Work out the finished part from the listing and answer in its coordinate system (mm). A direction names the side the tool comes from. Coordinates: 2 decimals unless noted, no trailing zeros. Write each loop counter-clockwise with the first axis right and the second up, starting at its lowest first coordinate (ties: lowest second). Pieces come first, ordered by that corner, then holes. Notation, with made-up numbers: (36, -15.5) - (75, -15.5) arc R18 cw to (75, 16.5) - close; hole circle Ø11 at (84.25, -9.5). An arc over 180 degrees is marked (long way). Use a Markdown table: item, result. Add a question column.
(1) For a pull along Y with two mould halves and no side action, classify faces 1 (the face through (2, -1.588, 2)), 2 (the face through (10.17, -2.35, 8.57)), 3 (the face through (-5.506, -2.37, -24.796)) as released by +Y, released by -Y, zero draft, split by the parting line, or undercut.
(2) Find the intervals of material crossed by line 1 (Z direction, x = 0, y = -3.4) (3 decimals); line 2 (Z direction, x = 0, y = -2) (3 decimals); line 3 (X direction, y = -0.5, z = -7), in increasing order. Write a range as from..to.
(3) Given pin 1 Ø1.6 at (x, y) = (1.5, -3) entering from +Z; pin 2 Ø2 at (y, z) = (-4, -18) entering from -X; pin 3 Ø7 at (x, z) = (-2.5, -2) entering from -Y, each flat-ended and moving along its own axis, determine where each tip first touches the part or whether it passes through.
(4) The part is cut by section D-D, the plane x = -14. Give the vertices of the cut face in (y, z) (1 decimal).
(5) The part is cut by section A-A, the plane x = 0. Give the vertices of the cut face in (y, z) (1 decimal).
(6) The part is cut by section C-C, the plane z = 15.24. Give the vertices of the cut face in (x, y) (1 decimal).
(7) The part is cut by section B-B, the plane z = 7.62. Give the vertices of the cut face in (x, y) (1 decimal).
(8) A tool of negligible diameter and unlimited length cuts with its end or side. For faces 4 (the face through (0, -3, -6.858)), 5 (the face through (24, -3.175, -10)), 6 (the face through (6, -4.762, -6)), from which of +Z, -Z, +X, -X, +Y, -Y can it reach the whole face along a straight path? Write none if from no direction.
from build123d import *

# Parameters (mm, degrees)
F0_R     = 26.67
F0_R_2   = 25.4
F1_DEPTH = 1.5875
F2_R     = 25.4
F3_DEPTH = 1.5875
F4_R     = 26.67
F4_R_2   = 25.4
F5_DEPTH = 1.5875
F6_R     = 1.905
F7_DEPTH = 25.4
F9_D     = 6.35


# Not quite as in the source:
# - a length typed as a fraction of an inch, garbled in the dataset ("3 / 203.2 mm" for 3/8 in), is restored


with BuildPart() as f1:
    # F0 (on Front) → F1 (new body)
    with BuildSketch(Plane.XZ):
        Circle(F0_R)
        Circle(F0_R_2, mode=Mode.SUBTRACT)
        Circle(F0_R_2)
        with BuildLine():
            ThreePointArc((3.9594681461, 6.858), (6.858, 3.9594681461), (7.9189362922, 0))
            ThreePointArc((7.9189362922, 0), (6.858, -3.9594681461), (3.9594681461, -6.858))
            ThreePointArc((3.9594681461, -6.858), (0, -7.9189362922), (-3.9594681461, -6.858))
            ThreePointArc((-3.9594681461, -6.858), (-6.858, -3.9594681461), (-7.9189362922, 0))
            ThreePointArc((-7.9189362922, 0), (-6.858, 3.9594681461), (-3.9594681461, 6.858))
            ThreePointArc((-3.9594681461, 6.858), (0, 7.9189362922), (3.9594681461, 6.858))
        make_face(mode=Mode.SUBTRACT)
        Polygon((3.9594681461, -6.858), (7.9189362922, 0), (3.9594681461, 6.858), (-3.9594681461, 6.858), (-7.9189362922, 0), (-3.9594681461, -6.858), align=None)
        with BuildLine():
            Line((-3.9594681461, 6.858), (3.9594681461, 6.858))
            ThreePointArc((3.9594681461, 6.858), (0, 7.9189362922), (-3.9594681461, 6.858))
        make_face()
        with BuildLine():
            Line((3.9594681461, 6.858), (7.9189362922, 0))
            ThreePointArc((7.9189362922, 0), (6.858, 3.9594681461), (3.9594681461, 6.858))
        make_face()
        with BuildLine():
            ThreePointArc((3.9594681461, -6.858), (6.858, -3.9594681461), (7.9189362922, 0))
            Line((7.9189362922, 0), (3.9594681461, -6.858))
        make_face()
        with BuildLine():
            ThreePointArc((-3.9594681461, -6.858), (0, -7.9189362922), (3.9594681461, -6.858))
            Line((3.9594681461, -6.858), (-3.9594681461, -6.858))
        make_face()
        with BuildLine():
            ThreePointArc((-7.9189362922, 0), (-6.858, -3.9594681461), (-3.9594681461, -6.858))
            Line((-3.9594681461, -6.858), (-7.9189362922, 0))
        make_face()
        with BuildLine():
            Line((-7.9189362922, 0), (-3.9594681461, 6.858))
            ThreePointArc((-3.9594681461, 6.858), (-6.858, 3.9594681461), (-7.9189362922, 0))
        make_face()
    extrude(amount=F1_DEPTH)

    # F2 (on face) → F3 (join)
    with BuildSketch(Plane.XZ.offset(1.5875)):
        Circle(F2_R)
        with BuildLine():
            ThreePointArc((3.9594681461, 6.858), (6.858, 3.9594681461), (7.9189362922, 0))
            ThreePointArc((7.9189362922, 0), (6.858, -3.9594681461), (3.9594681461, -6.858))
            ThreePointArc((3.9594681461, -6.858), (0, -7.9189362922), (-3.9594681461, -6.858))
            ThreePointArc((-3.9594681461, -6.858), (-6.858, -3.9594681461), (-7.9189362922, 0))
            ThreePointArc((-7.9189362922, 0), (-6.858, 3.9594681461), (-3.9594681461, 6.858))
            ThreePointArc((-3.9594681461, 6.858), (0, 7.9189362922), (3.9594681461, 6.858))
        make_face(mode=Mode.SUBTRACT)
        with BuildLine():
            Line((3.9594681461, 6.858), (7.9189362922, 0))
            ThreePointArc((7.9189362922, 0), (6.858, 3.9594681461), (3.9594681461, 6.858))
        make_face()
        with BuildLine():
            Line((-3.9594681461, 6.858), (3.9594681461, 6.858))
            ThreePointArc((3.9594681461, 6.858), (0, 7.9189362922), (-3.9594681461, 6.858))
        make_face()
        with BuildLine():
            Line((-7.9189362922, 0), (-3.9594681461, 6.858))
            ThreePointArc((-3.9594681461, 6.858), (-6.858, 3.9594681461), (-7.9189362922, 0))
        make_face()
        with BuildLine():
            ThreePointArc((-7.9189362922, 0), (-6.858, -3.9594681461), (-3.9594681461, -6.858))
            Line((-3.9594681461, -6.858), (-7.9189362922, 0))
        make_face()
        with BuildLine():
            ThreePointArc((-3.9594681461, -6.858), (0, -7.9189362922), (3.9594681461, -6.858))
            Line((3.9594681461, -6.858), (-3.9594681461, -6.858))
        make_face()
        with BuildLine():
            ThreePointArc((3.9594681461, -6.858), (6.858, -3.9594681461), (7.9189362922, 0))
            Line((7.9189362922, 0), (3.9594681461, -6.858))
        make_face()
    extrude(amount=F3_DEPTH)

    # F4 (on face) + F0 (on Front) → F5 (join)
    with BuildSketch(Plane.XZ.offset(3.175)):
        Circle(F4_R)
        Circle(F4_R_2, mode=Mode.SUBTRACT)
        Circle(F4_R_2)
        Polygon((7.9189362922, 0), (3.9594681461, -6.858), (-3.9594681461, -6.858), (-7.9189362922, 0), (-3.9594681461, 6.858), (3.9594681461, 6.858), align=None, mode=Mode.SUBTRACT)
    with BuildSketch(Plane.XZ):
        Circle(F0_R)
        Circle(F0_R_2, mode=Mode.SUBTRACT)
    extrude(amount=F5_DEPTH)

    # F6 (on face) → F7 (cut)
    with BuildSketch(Plane.XZ.offset(1.5875)):
        Circle(F6_R)
    extrude(amount=-F7_DEPTH, mode=Mode.SUBTRACT)

    # F9 (through all)
    with Locations(Plane.XZ.offset(4.7625)):
        with Locations((0, 15.24), (0, -15.24), (-13.1982271537, -7.62), (-13.1982271537, 7.62), (13.1982271537, 7.62), (13.1982271537, -7.62)):
            Hole(F9_D / 2)


solid = f1.part
Model answer:
| question | item | result |
|---|---|---|
| 1 | face 1 | released by -Y |
| 1 | face 2 | zero draft |
| 1 | face 3 | undercut |
| 2 | line 1 | -26.67..-18.415, -12.065..-6.858, 6.858..12.065, 18.415..26.67 |
| 2 | line 2 | -25.4..-18.415, -12.065..-6.858, 6.858..12.065, 18.415..25.4 |
| 2 | line 3 | -25.73..-16.31, -10.08..10.08, 16.31..25.73 |
| 3 | pin 1 | z = 26.66 |
| 3 | pin 2 | x = -20.55 |
| 3 | pin 3 | y = -1.59 |
| 4 | outline | (-4.8, -22.7) - (-3.2, -22.7) - (-3.2, -21.2) - (-1.6, -21.2) - (-1.6, -22.7) - (0, -22.7) - (0, -10.7) - (-4.8, -10.7) - close; (-4.8, -4.5) - (0, -4.5) - (0, 4.5) - (-4.8, 4.5) - close; (-4.8, 10.7) - (0, 10.7) - (0, 22.7) - (-1.6, 22.7) - (-1.6, 21.2) - (-3.2, 21.2) - (-3.2, 22.7) - (-4.8, 22.7) - close |
| 5 | outline | (-4.8, -26.7) - (-3.2, -26.7) - (-3.2, -25.4) - (-1.6, -25.4) - (-1.6, -26.7) - (0, -26.7) - (0, -18.4) - (-4.8, -18.4) - close; (-4.8, -12.1) - (0, -12.1) - (0, -1.9) - (-1.6, -1.9) - (-1.6, -6.9) - (-4.8, -6.9) - close; (-4.8, 6.9) - (-1.6, 6.9) - (-1.6, 1.9) - (0, 1.9) - (0, 12.1) - (-4.8, 12.1) - close; (-4.8, 18.4) - (0, 18.4) - (0, 26.7) - (-1.6, 26.7) - (-1.6, 25.4) - (-3.2, 25.4) - (-3.2, 26.7) - (-4.8, 26.7) - close |
| 6 | outline | (-21.9, -4.8) - (-3.2, -4.8) - (-3.2, 0) - (-21.9, 0) - (-21.9, -1.6) - (-20.3, -1.6) - (-20.3, -3.2) - (-21.9, -3.2) - close; (3.2, -4.8) - (21.9, -4.8) - (21.9, -3.2) - (20.3, -3.2) - (20.3, -1.6) - (21.9, -1.6) - (21.9, 0) - (3.2, 0) - close |
| 7 | outline | (-25.6, -4.8) - (-16.4, -4.8) - (-16.4, 0) - (-25.6, 0) - (-25.6, -1.6) - (-24.2, -1.6) - (-24.2, -3.2) - (-25.6, -3.2) - close; (-10, -4.8) - (10, -4.8) - (10, 0) - (-10, 0) - close; (16.4, -4.8) - (25.6, -4.8) - (25.6, -3.2) - (24.2, -3.2) - (24.2, -1.6) - (25.6, -1.6) - (25.6, 0) - (16.4, 0) - close |
| 8 | face 4 | -Y |
| 8 | face 5 | none |
| 8 | face 6 | +Z, -Z, +X, -X, -Y |
